The model under review builds one solid part; all positions refer to its coordinate system, in mm. Face numbers are marked on the shaded views. A direction names the side the tool comes from. Give positions to 0.01 mm unless a question says otherwise; leave off trailing zeros. Order: outer loops, then holes, each group sorted by start corner. A loop starts at its lowest first (then second) coordinate and runs counter-clockwise, first axis right, second up. Notation, with made-up numbers: (-14, 68.25) - (13, 68.25) arc R16 ccw to (13, 98.25) - close; hole circle Ø2 at (2.25, 32). An arc over 180 degrees is marked (long way). Write item = value, one per line. Start each with the question number.
1. Machinability: for the marked faces 1 and 2, which of the approach directions +Z, -Z, +X, -X, +Y, -Y give a long, thin tool a straight path to every point of the face, cutting with its end or side? Answer none if there is none.
2. For P1, Ø3, axis at x = -1.5, y = 5.5, coming from the +Z side; P2, Ø1.5, axis at x = 0, y = 3, coming from the -Z side, all flat-tipped, find the tip position at first contact; note any pin that passes through.
3. We need section C-C, the plane y = 5.5. Give the boundary of the cut face in (x, z).
4. We need section A-A, the plane x = 0. Give the boundary of the cut face in (y, z), and give its area (3 significant figures).
5. Wall thickness on probe 1 along X at (y, z) = (1.95, 0); probe 2 along X at (y, z) = (-0.6, 0); probe 3 along Y at (x, z) = (7, -3): over which ranges is each line inside the solid? List them lowest first.
6. We need section B-B, the plane z = 0. Give the boundary of the cut face in (x, y).
7. Mouldability with a two-part tool opening along Z and no side actions: class the marked faces 3, 4, 5 and 6 as pulls with the +Z half, pulls with the -Z half, needs draft (parallel to the pull), parting line crosses it, or undercut.
8. We need section D-D, the plane y = -0.25. Give the boundary of the cut face in (x, z), and give its area (3 significant figures).
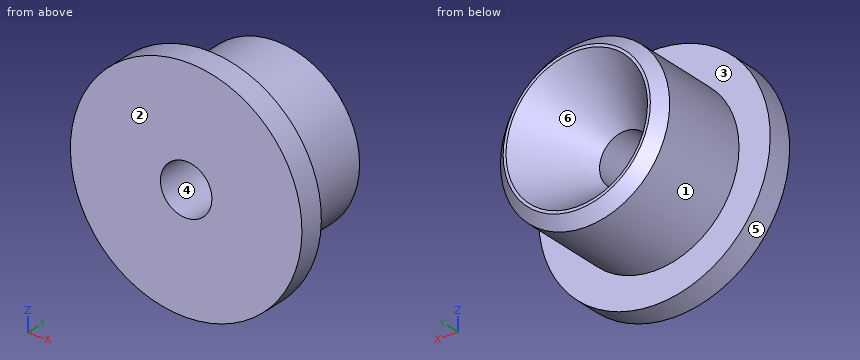
from build123d import *


# Read off the part's stored shape, not the designer's step: G1/4 Straight Pipe Tapped Thread Stud1
with BuildPart() as part:
    # Sketch1 → Revolve1 (revolve)
    with BuildSketch(Plane.XY, mode=Mode.PRIVATE) as revolve1_sk:
        Polygon((7, 0), (2, 0), (2, 3), (5.5, 8), (7, 8), align=None)
        Polygon((7, 0), (2, 0), (2, -2), (9, -2), (9, 0), align=None)
    revolve(revolve1_sk.sketch.rotate(Axis((0, 0, 0), (0, 1, 0)), 90), axis=Axis((0, 0, 0), (0, 1, 0)))

    # G1/4 Straight Pipe Tapped Thread Stud1 o → G1/4 Straight Pipe Tapped Thread Stud1 (revolve, cut)
    with BuildSketch(Plane.XY):
        Polygon((7, 8), (5.7225, 8), (6.5785, 7.144), (6.5785, 0), (7, 0), align=None)
    revolve(axis=Axis((0, 0, 0), (0, 1, 0)), mode=Mode.SUBTRACT)


solid = part.part
Model answer:
q1.face_1 = +Y
q1.face_2 = +Z, -Z, +X, -X, -Y
q2.P1 = 6.58
q2.P2 = -6.58
q3.outline = circle Ø13.16 at (0, 0); hole circle Ø7.5 at (0, 0)
q4.outline = (-2, -9) - (0, -9) - (0, -6.58) - (7.14, -6.58) - (8, -5.72) - (8, -5.5) - (3, -2) - (-2, -2) - close; (-2, 2) - (3, 2) - (8, 5.5) - (8, 5.72) - (7.14, 6.58) - (0, 6.58) - (0, 9) - (-2, 9) - close
q4.area = 83.0 mm2
q5.probe_1 = -6.58 to -2, 2 to 6.58
q5.probe_2 = -9 to -2, 2 to 9
q5.probe_3 = -2 to 0
q6.outline = (-9, -2) - (-2, -2) - (-2, 3) - (-5.5, 8) - (-5.72, 8) - (-6.58, 7.14) - (-6.58, 0) - (-9, 0) - close; (2, -2) - (9, -2) - (9, 0) - (6.58, 0) - (6.58, 7.14) - (5.72, 8) - (5.5, 8) - (2, 3) - close
q7.face_3 = needs draft
q7.face_4 = undercut
q7.face_5 = parting line crosses it
q7.face_6 = undercut
q8.outline = circle Ø18 at (0, 0); hole circle Ø4 at (0, 0)
q8.area = 242 mm2
